```python
from build123d import *

# Parameters (mm, degrees)
BOSS_EXTRUDE1_DEPTH      = 4
BOSS_EXTRUDE2_DEPTH      = 0.01
BOSS_EXTRUDE2_DEPTH_BACK = 32.01
SKETCH4_R                = 4.5
CUT_EXTRUDE1_DEPTH       = 23
CUT_EXTRUDE2_DEPTH       = 217.234410074
CUT_EXTRUDE2_DEPTH_BACK  = 217.234410074
SKETCH5_R                = 4
SKETCH6_R                = 4
BOSS_EXTRUDE3_DEPTH      = 10
FILLET1_R                = 3
BOSS_EXTRUDE6_DEPTH      = 24


with BuildPart() as part:
    # Sketch2 → Boss-Extrude1 (new body)
    with BuildSketch(Plane.XY.offset(16)):
        with BuildLine():
            Line((10, 0), (34.214158147, 41.940152173))
            ThreePointArc((34.214158147, 41.940152173), (41.467493607, 49.878296982), (51.384329922, 54.035384403))
            Line((51.384329922, 54.035384403), (150, 72))
            Line((150, 72), (150, 28))
            Line((150, 28), (104.559799809, 23.906962122))
            ThreePointArc((104.559799809, 23.906962122), (95.230440402, 21.168208391), (87.651490086, 15.077458761))
            Line((87.651490086, 15.077458761), (75, 0))
            Line((75, 0), (10, 0))
        make_face()
    extrude(amount=-BOSS_EXTRUDE1_DEPTH)


with BuildPart() as body_2:
    # Mirror2: mirrored copy
    add(part.part.mirror(Plane.XY))


with BuildPart() as part_1:
    add(part.part)

    add(body_2.part)  # Boss-Extrude2 merges body 2
    # Sketch3 → Boss-Extrude2 (add, two sides: drawn at the far end of the back side and taken through both)
    with BuildSketch(Plane.XY.offset(16).offset(-BOSS_EXTRUDE2_DEPTH_BACK)):
        with BuildLine():
            Line((189.966629547, 51), (210, 51))
            Line((210, 51), (210, 72))
            Line((210, 72), (150, 72))
            Line((150, 72), (150, 28))
            Line((150, 28), (210, 28))
            Line((210, 28), (210, 49))
            Line((210, 49), (189.966629547, 49))
            ThreePointArc((189.966629547, 49), (160, 50), (189.966629547, 51))
        make_face()
    extrude(amount=BOSS_EXTRUDE2_DEPTH + BOSS_EXTRUDE2_DEPTH_BACK)

    # Sketch4 → Cut-Extrude1 (cut)
    with BuildSketch(Plane(origin=(0, 72, 0), x_dir=(1, 0, 0), z_dir=(0, 1, 0))):
        with Locations(Location((200, 0.005, 0), (0, 0, 270))):
            Circle(SKETCH4_R)
    extrude(amount=-CUT_EXTRUDE1_DEPTH, mode=Mode.SUBTRACT)

    # Sketch5 → Cut-Extrude2 (cut, two sides: drawn at the far end of the back side and taken through both)
    with BuildSketch(Plane(origin=(0, 49, 0), x_dir=(1, 0, 0), z_dir=(0, 1, 0)).offset(-CUT_EXTRUDE2_DEPTH_BACK)):
        with Locations(Location((200, 0.005, 0), (0, 0, 180))):
            Circle(SKETCH5_R)
    extrude(amount=CUT_EXTRUDE2_DEPTH + CUT_EXTRUDE2_DEPTH_BACK, mode=Mode.SUBTRACT)

    # Sketch6 → Boss-Extrude3 (add)
    with BuildSketch(Plane(origin=(0, 0, 0), x_dir=(1, 0, 0), z_dir=(0, 1, 0))):
        with BuildLine():
            Line((-7.870410355, 6.169006472), (3.703671716, 20.935205177))
            ThreePointArc((3.703671716, 20.935205177), (5.655280169, 22.717396042), (8.081072691, 23.766448222))
            Line((8.081072691, 23.766448222), (72.601340863, 39.708060277))
            ThreePointArc((72.601340863, 39.708060277), (81.164957771, 37.873582138), (85, 30))
            Line((85, 30), (85, -30))
            ThreePointArc((85, -30), (81.164957771, -37.873582138), (72.601340863, -39.708060277))
            Line((72.601340863, -39.708060277), (8.081072691, -23.766448222))
            ThreePointArc((8.081072691, -23.766448222), (5.655280169, -22.717396042), (3.703671716, -20.935205177))
            Line((3.703671716, -20.935205177), (-7.870410355, -6.169006472))
            ThreePointArc((-7.870410355, -6.169006472), (-10, 0), (-7.870410355, 6.169006472))
        make_face()
        with Locations(Location((75, 30, 0), (0, 0, 270))):
            Circle(SKETCH6_R, mode=Mode.SUBTRACT)
        with Locations(Location((75, -30, 0), (0, 0, 270))):
            Circle(SKETCH6_R, mode=Mode.SUBTRACT)
        with Locations(Location((0, 0, 0), (0, 0, 270))):
            Circle(SKETCH6_R, mode=Mode.SUBTRACT)
    extrude(amount=-BOSS_EXTRUDE3_DEPTH)

    # Fillet1
    fillet1_edges = [part_1.edges().sort_by_distance(p)[0] for p in [
        (5.655280169, 0, -22.717396042),
        (-2.083369319, 0, -13.552105825),
        (-10, 0, 0),
        (-2.083369319, 0, 13.552105825),
        (5.655280169, 0, 22.717396042),
        (40.341206777, 0, 31.73725425),
        (81.164957771, 0, 37.873582138),
        (85, 0, 0),
        (81.164957771, 0, -37.873582138),
        (40.341206777, 0, -31.73725425),
        (5.655280169, -10, -22.717396042),
        (40.341206777, -10, -31.73725425),
        (81.164957771, -10, -37.873582138),
        (85, -10, 0),
        (81.164957771, -10, 37.873582138),
        (40.341206777, -10, 31.73725425),
        (5.655280169, -10, 22.717396042),
        (-2.083369319, -10, 13.552105825),
        (-10, -10, 0),
        (-2.083369319, -10, -13.552105825),
    ]]
    fillet(fillet1_edges, radius=FILLET1_R)

    # Sketch9 → Boss-Extrude6 (add)
    with BuildSketch(Plane(origin=(0, 0, 12), x_dir=(-1, 0, 0), z_dir=(0, 0, -1))):
        with BuildLine():
            Line((-75, 0), (-68.975115859, 0))
            Line((-68.975115859, 0), (-37.662167154, 46.576791386))
            ThreePointArc((-37.662167154, 46.576791386), (-39.481454935, 48.323643003), (-41.467493607, 49.878296982))
            Line((-41.467493607, 49.878296982), (-72.096679368, 4.31857634))
            Line((-72.096679368, 4.31857634), (-125.078747354, 67.460146206))
            Line((-125.078747354, 67.460146206), (-132.783511462, 68.863707378))
            Line((-132.783511462, 68.863707378), (-150, 38.210356026))
            Line((-150, 38.210356026), (-150, 28))
            Line((-150, 28), (-129.348247033, 64.769718653))
            Line((-129.348247033, 64.769718653), (-75, 0))
        make_face()
    extrude(amount=BOSS_EXTRUDE6_DEPTH)


solid = part_1.part
```
The listing builds one solid part. Answer for the finished solid, in the listing's coordinates (mm). A direction names the side the tool comes from. Give positions to 0.01 mm unless a question says otherwise; leave off trailing zeros. Order: outer loops, then holes, each group sorted by start corner. A loop starts at its lowest first (then second) coordinate and runs counter-clockwise, first axis right, second up.
Item 1: The part is cut by section D-D, the plane z = 2. Count the separate pieces of the cut face and the enclosed holes in it, and give its area (3 significant figures).
From the geometry:
separate pieces: 4
enclosed holes: 0
area: 3,360 mm2
Item 2: Which of the six approach directions +Z, -Z, +X, -X, +Y, -Y give full straight-line access (tool end or side, diameter ignored) to faces 5 (the face through (126, 38, 12)), 6 (the face through (75, 43, -12)), 7 (the face through (40, 13, -12)), 8 (the face through (81, 37, 16))?
From the geometry:
face 5: -Y
face 6: +Y
face 7: -X
face 8: +Z, +X, -X, +Y
Item 3: Find the intervals of material crossed by probe 1 along Z at (x, y) = (53, 52); probe 2 along X at (y, z) = (-5.25, 0); probe 3 along X at (y, z) = (60, -9), in increasing order.
From the geometry:
probe 1: z = -16 to -12, 12 to 16
probe 2: x = -10 to -4, 4 to 85
probe 3: x = 118.82 to 125.35, 132.03 to 137.76, 150 to 163.82, 186.18 to 210
Item 4: The part is cut by section C-C, the plane y = 21.5. Give the vertices of the cut face in (x, z), and give its area (3 significant figures).
From the geometry:
outline: (22.41, -16) - (95.89, -16) - (95.89, -12) - (93.04, -12) - (93.04, 12) - (95.89, 12) - (95.89, 16) - (22.41, 16) - (22.41, 12) - (54.52, 12) - (54.52, -12) - (22.41, -12) - close; hole (60.55, -12) - (86.51, -12) - (86.51, 12) - (60.55, 12) - close
area: 889 mm2
Item 5: The part is cut by section A-A, the plane x = 175. Give the vertices of the cut face in (y, z), and give its area (3 significant figures).
From the geometry:
outline: (28, -16.01) - (35, -16.01) - (35, 16.01) - (28, 16.01) - close; (65, -16.01) - (72, -16.01) - (72, 16.01) - (65, 16.01) - close
area: 448 mm2
Item 6: The part is cut by section B-B, the plane x = 200. Give the vertices of the cut face in (y, z) (3 decimals).
From the geometry:
outline: (28, -16.01) - (49, -16.01) - (49, -4.005) - (28, -4.005) - close; (28, 3.995) - (49, 3.995) - (49, 16.01) - (28, 16.01) - close; (51, -16.01) - (72, -16.01) - (72, -4.505) - (51, -4.505) - close; (51, 4.495) - (72, 4.495) - (72, 16.01) - (51, 16.01) - close
Item 7: Given pin 1 Ø19 at (y, z) = (49, -3.5) entering from -X; pin 2 Ø2 at (x, y) = (100.5, 63) entering from -Z; pin 3 Ø10 at (x, z) = (146.5, 9) entering from -Y; pin 4 Ø18 at (x, y) = (175, 50) entering from +Z, each flat-ended and moving along its own axis, determine where each tip first touches the part or whether it passes through.
From the geometry:
pin 1: stops at x = 36.11
pin 2: stops at z = -16
pin 3: stops at y = 27.32
pin 4: passes through
Item 8: For a pull along X with two mould halves and no side action, classify faces 1 (the face through (53.54, 22.96, 0.17)), 2 (the face through (-3.905, -4.93, -0.867)), 3 (the face through (145, 59, -12)), 4 (the face through (210, 38, 0)) as pulls with the +X half, pulls with the -X half, needs draft (parallel to the pull), parting line crosses it, or undercut.
From the geometry:
face 1: pulls with the -X half
face 2: undercut
face 3: undercut
face 4: pulls with the +X half
